```python
from build123d import *

# Parameters (mm, degrees)
F0_R     = 7.6617406775
F2_R     = 6
F4_R     = 2
F5_R     = 4.7899887375
F6_DEPTH = 2
F8_R     = 5.1
F9_DEPTH = 4


# Not quite as in the source:
# - a fillet or chamfer that OpenCascade refuses, or shapes differently, is made with other operations: its cross-section is extruded or revolved along the edge and cut away or added


with BuildPart() as f3:
    # F0 (on Top) → F3 section 0
    with BuildSketch(Plane.XY):
        Circle(F0_R)
    # F2 (on offset) → F3 section 1
    with BuildSketch(Plane.XY.offset(7)):
        Circle(F2_R)
    loft()

    # F4
    f4_edges = [f3.edges().sort_by_distance(p)[0] for p in [
        (-7.661741, 0, 0),
    ]]
    fillet(f4_edges, radius=F4_R)

    # F5 (on face) → F6 (join)
    with BuildSketch(Plane(origin=(0, 0, 0), x_dir=(1, 0, 0), z_dir=(0, 0, -1))):
        Circle(F5_R)
    extrude(amount=F6_DEPTH)

    # F7: fillet of radius 5 on 1 edges, made by hand

    # F7_s1 → F7_t2 (revolve, cut)
    with BuildSketch(Plane.XZ):
        with BuildLine():
            ThreePointArc((4.7899887375, 0), (3.026056715, -1.472135955), (0.7899887375, -2))
            Line((0.7899887375, -2), (4.7899887375, -2))
            Line((4.7899887375, -2), (4.7899887375, 0))
        make_face()
    revolve(axis=Axis((0, 0, -2), (0, 0, -1)), mode=Mode.SUBTRACT)

    # F8 (on face) → F9 (cut)
    with BuildSketch(Plane.XY.offset(7)):
        Circle(F8_R)
    extrude(amount=-F9_DEPTH, mode=Mode.SUBTRACT)


solid = f3.part
```
Part model, mm, in its own coordinate system. A direction names the side the tool comes from. Coordinates: 2 decimals unless noted, no trailing zeros. Loops run counter-clockwise (first coordinate to the right, second up) from the corner with the lowest first, then second, coordinate; pieces in that order, holes last. Notation, with made-up numbers: (61, -27) - (86, -27) arc R10 cw to (86, -23) - close; hole circle Ø3 at (86, 79). An arc over 180 degrees is marked (long way). Write item = value, one per line. Start each with the question number.
Item 1: Flat gauge pins, fed straight in: pin 1 Ø3 at (y, z) = (-3.5, 1) entering from -X; pin 2 Ø8 at (x, y) = (1, -1.5) entering from +Z; pin 3 Ø3 at (x, y) = (2.5, 1) entering from -Z; pin 4 Ø3 at (x, z) = (1.5, 5.5) entering from -Y. Where does each tip first touch, or does it go through?
Item 2: Cut at A-A, the plane z = 2. Give the cut face in (x, y).
Item 3: Cut at B-B, the plane z = 3.5. Give the cut face in (x, y), and give its area (3 significant figures).
Item 4: Wall check: L1, parallel to Y at x = 3.5, z = 6.75; L2, parallel to Y at x = 0, z = 4.3; L3, parallel to Z at x = 5, y = 0.25. Give the ranges that are in metal, low to high. Write a range as from..to.
Item 5: Mould opens along X. For faces 1 (the cylindrical face through (2.4, -4.5, 5)), 2 (the flat face through (0, 0, -2)), 3 (the conical face through (-0.8, 6.12, 6.28)) say: released by +X, released by -X, zero draft, split by the parting line, or undercut.
Item 6: Cut at C-C, the plane z = 1. Give the cut face in (x, y).
Item 7: 3-axis set-ups, long thin cutter, end or side, ignore diameter. For faces 4 (the flat face through (0, 0, 3)), 5 (the flat face through (-2, -5, 7)): which of +Z, -Z, +X, -X, +Y, -Y reach the whole face in a straight line?
The answers:
q1.pin_1 = -6.77
q1.pin_2 = 7
q1.pin_3 = -1.98
q1.pin_4 = -6.62
q2.outline = circle Ø14.26 at (0, 0)
q3.outline = circle Ø13.66 at (0, 0); hole circle Ø10.2 at (0, 0)
q3.area = 64.9 mm2
q4.L1 = -4.95..-3.71, 3.71..4.95
q4.L2 = -6.64..-5.1, 5.1..6.64
q4.L3 = 0..3
q5.face_1 = undercut
q5.face_2 = zero draft
q5.face_3 = split by the parting line
q6.outline = circle Ø13.73 at (0, 0)
q7.face_4 = +Z
q7.face_5 = +Z, +X, -X, +Y, -Y
